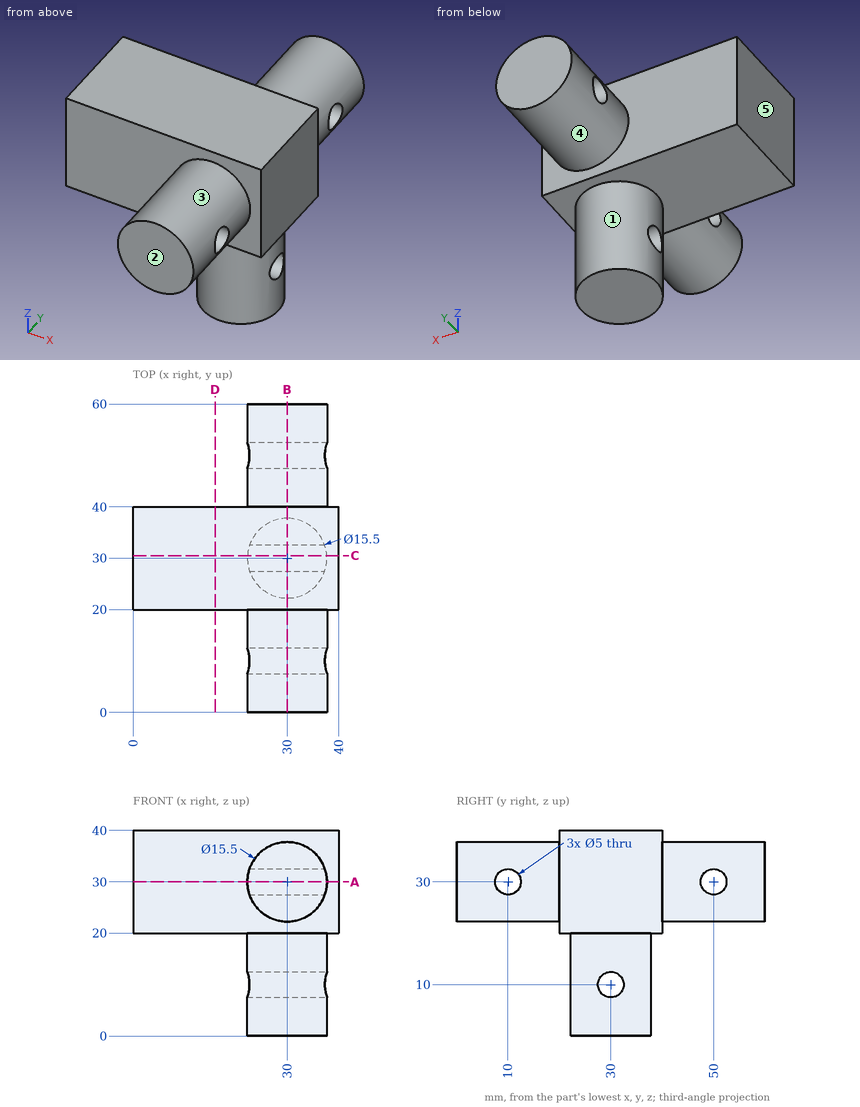
Here's the drawing with two shaded views (mm, measured from the low corner). I have some questions. A direction names the side the tool comes from. Give positions to 0.01 mm unless a question says otherwise; leave off trailing zeros. Loops run counter-clockwise (first coordinate to the right, second up) from the corner with the lowest first, then second, coordinate; pieces in that order, holes last. Notation, with made-up numbers: M 64,22.25 L 73,22.25 A36 ccw 73,56.25 Z; hole C 66.5,-13.5 d3. An arc over 180 degrees is marked long. One line per item, written item: value.
1) On a 3-axis mill with a long thin cutter (end or side, diameter ignored), from which of +Z, -Z, +X, -X, +Y, -Y can I reach the whole of each face in a straight line? I mean the marked faces 1, 2, 3, 4 and 5. Say none if no direction works.
Geometry check:
face 1: -Z
face 2: +Z, -Z, +X, -X, -Y
face 3: -Y
face 4: +Y
face 5: +Z, -Z, -X, +Y, -Y
2) Imagine slicing it at C-C on y = 30.5. Write out the boundary of the cut face in (x, z), and give its area (3 significant figures).
Geometry check:
outline: M 0,20 L 22.27,20 L 22.27,12.45 L 37.73,12.45 L 37.73,20 L 40,20 L 40,40 L 0,40 Z; M 22.27,0 L 37.73,0 L 37.73,7.55 L 22.27,7.55 Z
area: 1,030 mm²
3) I'm going to push flat-ended pins straight in: pin 1 (6 mm diameter, centred on y = 21, z = 15.5, fed in from -X); pin 2 (4 mm diameter, centred on x = 12, z = 20.5, fed in from +Y); pin 3 (5 mm diameter, centred on x = 31, z = 5, fed in from +Y). Where does each tip first touch, or does it pass through?
Geometry check:
pin 1: stops at x = 25.09
pin 2: stops at y = 40
pin 3: stops at y = 37.75
4) Imagine slicing it at B-B on x = 30. Write out the boundary of the cut face in (y, z), and give its area (3 significant figures).
Geometry check:
outline: M 0,22.25 L 20,22.25 L 20,20 L 22.25,20 L 22.25,0 L 37.75,0 L 37.75,20 L 40,20 L 40,22.25 L 60,22.25 L 60,37.75 L 40,37.75 L 40,40 L 20,40 L 20,37.75 L 0,37.75 Z; hole C 10,30 d5; hole C 30,10 d5; hole C 50,30 d5
area: 1,270 mm²
5) Imagine slicing it at D-D on x = 16. Write out the boundary of the cut face in (y, z), and give its area (3 significant figures).
Geometry check:
outline: M 20,20 L 40,20 L 40,40 L 20,40 Z
area: 400 mm²
6) Imagine slicing it at A-A on z = 30. Write out the boundary of the cut face in (x, y), and give its area (4 significant figures).
Geometry check:
outline: M 0,20 L 22.25,20 L 22.25,12.5 L 37.75,12.5 L 37.75,20 L 40,20 L 40,40 L 37.75,40 L 37.75,47.5 L 22.25,47.5 L 22.25,40 L 0,40 Z; M 22.25,0 L 37.75,0 L 37.75,7.5 L 22.25,7.5 Z; M 22.25,52.5 L 37.75,52.5 L 37.75,60 L 22.25,60 Z
area: 1,265 mm²
7) Please list where these lines run through material, in increasing order: line 1 (Z direction, x = 29, y = 30); line 2 (Z direction, x = 29.5, y = 50); line 3 (Z direction, x = 21.5, y = 39).
Geometry check:
line 1: z = 0 to 7.5, 12.5 to 40
line 2: z = 22.27 to 27.5, 32.5 to 37.73
line 3: z = 20 to 40
